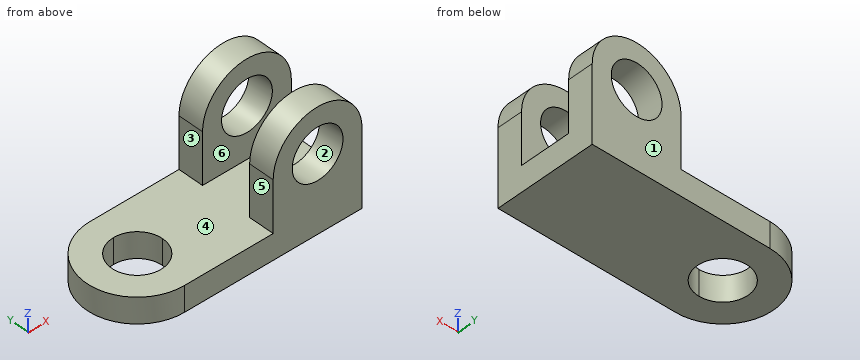
from build123d import *

# Parameters (mm, degrees)
F1_DEPTH  = 12.7
F2_DEPTH  = 12.7
F3_W      = 44.45
F3_H      = 12.7
F4_DEPTH  = 25.4
F6_DEPTH  = 12.7
F7_R      = 12.7
F8_DEPTH  = 25.4
F9_DEPTH  = 25.4
F11_DEPTH = 12.7
F12_R     = 12.7
F13_DEPTH = 25.4


with BuildPart() as f1:
    # F0 (on Top) → F1 (new body)
    with BuildSketch(Plane.XY):
        with BuildLine():
            ThreePointArc((-38.464964, 3.526151), (-63.864964, -21.873849), (-38.464964, -47.273849))
            Line((-38.464964, -47.273849), (-38.464964, -34.573849))
            ThreePointArc((-38.464964, -34.573849), (-51.164964, -21.873849), (-38.464964, -9.173849))
            Line((-38.464964, -9.173849), (-38.464964, 3.526151))
        make_face()
    extrude(amount=F1_DEPTH)

    # F0 (on Top) → F2 (join)
    with BuildSketch(Plane.XY):
        with BuildLine():
            Line((-38.464964, -47.273849), (50.435036, -47.273849))
            Line((50.435036, -47.273849), (50.435036, 3.526151))
            Line((50.435036, 3.526151), (-38.464964, 3.526151))
            Line((-38.464964, 3.526151), (-38.464964, -9.173849))
            ThreePointArc((-38.464964, -9.173849), (-29.484708, -12.893592), (-25.764964, -21.873849))
            ThreePointArc((-25.764964, -21.873849), (-29.484708, -30.854105), (-38.464964, -34.573849))
            Line((-38.464964, -34.573849), (-38.464964, -47.273849))
        make_face()
    extrude(amount=F2_DEPTH)

    # F3 (on face) → F4 (join)
    with BuildSketch(Plane.XY.offset(12.7)):
        with Locations((28.210036, -40.923849)):
            Rectangle(F3_W, F3_H)
    extrude(amount=F4_DEPTH)

    # F5 (on face) → F6 (join)
    with BuildSketch(Plane.XZ.offset(47.273849)):
        with BuildLine():
            Line((5.985036, 38.1), (50.435036, 38.1))
            ThreePointArc((50.435036, 38.1), (28.210036, 60.325), (5.985036, 38.1))
        make_face()
    extrude(amount=-F6_DEPTH)

    # F7 (on face) → F8 (cut)
    with BuildSketch(Plane.XZ.offset(47.273849)):
        with Locations((28.210036, 38.1)):
            Circle(F7_R)
    extrude(amount=-F8_DEPTH, mode=Mode.SUBTRACT)

    # F3 (on face) → F9 (join)
    with BuildSketch(Plane.XY.offset(12.7)):
        with Locations((28.210036, -2.823849)):
            Rectangle(F3_W, F3_H)
    extrude(amount=F9_DEPTH)

    # F10 (on face) → F11 (join)
    with BuildSketch(Plane(origin=(0, 3.526151, 0), x_dir=(-1, 0, 0), z_dir=(0, 1, 0))):
        with BuildLine():
            Line((-50.435036, 38.1), (-5.985036, 38.1))
            ThreePointArc((-5.985036, 38.1), (-28.210036, 60.325), (-50.435036, 38.1))
        make_face()
    extrude(amount=-F11_DEPTH)

    # F12 (on face) → F13 (cut)
    with BuildSketch(Plane(origin=(0, 3.526151, 0), x_dir=(-1, 0, 0), z_dir=(0, 1, 0))):
        with Locations((-28.210036, 38.1)):
            Circle(F12_R)
    extrude(amount=-F13_DEPTH, mode=Mode.SUBTRACT)


solid = f1.part
Read the model definition and answer for the solid it produces. Units are mm, in the model's axes. Face numbers are marked on the shaded views. A direction names the side the tool comes from. Coordinates: 2 decimals unless noted, no trailing zeros. Loops run counter-clockwise (first coordinate to the right, second up) from the corner with the lowest first, then second, coordinate; pieces in that order, holes last. Notation, with made-up numbers: (44.5, 14.25) -> (65.5, 14.25) arc R26 cw to (65.5, 49.25) -> close; hole circle Ø6 at (-22, -18). An arc over 180 degrees is marked (long way). Answer in a Markdown table with one row per item.
Item 1: For a pull along X with two mould halves and no side action, classify the marked faces 1, 2 and 3 as released by +X, released by -X, zero draft, split by the parting line, or undercut.
Returned:
| item | result |
|---|---|
| face 1 | zero draft |
| face 2 | undercut |
| face 3 | released by -X |
Item 2: For the marked faces 4, 5 and 6, determine the directions among +Z, -Z, +X, -X, +Y, -Y from which every point of the face is accessible in a straight line to the end or side of a thin tool.
Returned:
| item | result |
|---|---|
| face 4 | +Z, -X |
| face 5 | +Z, -X, +Y, -Y |
| face 6 | +Z, +X, -X |
Item 3: A cutting plane is placed at D-D on x = 9. Determine the outline of the cut face in (y, z), plus the area to 3 significant figures.
Returned:
| item | result |
|---|---|
| outline | (-47.27, 0) -> (3.53, 0) -> (3.53, 49.28) -> (-9.17, 49.28) -> (-9.17, 12.7) -> (-34.57, 12.7) -> (-34.57, 49.28) -> (-47.27, 49.28) -> close |
| area | 1,570 mm^2 |
Item 4: A cutting plane is placed at A-A on z = 21. Determine the outline of the cut face in (x, y), plus the area to 3 significant figures.
Returned:
| item | result |
|---|---|
| outline | (5.99, -47.27) -> (50.44, -47.27) -> (50.44, -34.57) -> (5.99, -34.57) -> close; (5.99, -9.17) -> (50.44, -9.17) -> (50.44, 3.53) -> (5.99, 3.53) -> close |
| area | 1,130 mm^2 |
Item 5: A cutting plane is placed at B-B on x = -27.5. Determine the outline of the cut face in (y, z), plus the area to 3 significant figures.
Returned:
| item | result |
|---|---|
| outline | (-47.27, 0) -> (-28.28, 0) -> (-28.28, 12.7) -> (-47.27, 12.7) -> close; (-15.47, 0) -> (3.53, 0) -> (3.53, 12.7) -> (-15.47, 12.7) -> close |
| area | 482 mm^2 |
Item 6: Straight lines are drawn through the part: line 1 along Y through (x, z) = (45.5, 25); line 2 along X through (y, z) = (-39, 38); line 3 along Z through (x, y) = (-1, -42.5). For each, find the intervals that lie inside material, in ascending order. Write a range as [from, to].
Returned:
| item | result |
|---|---|
| line 1 | y = [-47.27, -34.57], [-9.17, 3.53] |
| line 2 | x = [5.99, 15.51], [40.91, 50.44] |
| line 3 | z = [0, 12.7] |
Item 7: A cutting plane is placed at C-C on z = 39.5. Determine the outline of the cut face in (x, y).
Returned:
| item | result |
|---|---|
| outline | (6.03, -47.27) -> (15.59, -47.27) -> (15.59, -34.57) -> (6.03, -34.57) -> close; (6.03, -9.17) -> (15.59, -9.17) -> (15.59, 3.53) -> (6.03, 3.53) -> close; (40.83, -47.27) -> (50.39, -47.27) -> (50.39, -34.57) -> (40.83, -34.57) -> close; (40.83, -9.17) -> (50.39, -9.17) -> (50.39, 3.53) -> (40.83, 3.53) -> close |
Item 8: Each of these flat-tipped pins is pushed along its axis until it touches: P1, Ø1.5, axis at x = 5.5, z = 21, coming from the +Y side; P2, Ø3, axis at y = -33.5, z = 44, coming from the +X side; P3, Ø6.5, axis at y = -43.5, z = 23.5, coming from the -X side; P4, Ø4, axis at y = -34, z = 9, coming from the -X side. Where does it stop, or does it pass through?
Returned:
| item | result |
|---|---|
| P1 | stops at y = 3.53 |
| P2 | stops at x = 49.9 |
| P3 | stops at x = 5.99 |
| P4 | stops at x = -61.76 |
